```python
from build123d import *

# Parameters (mm, degrees)
BOSS_EXTRUDE1_DEPTH             = 12.7
F_43_0_089_DIAMETER_HOLE1_D     = 2.2606
F_43_0_089_DIAMETER_HOLE1_DEPTH = 25.4
F_43_0_089_DIAMETER_HOLE1_TIP   = 0.679152758
F_43_0_089_DIAMETER_HOLE2_D     = 2.2606
F_43_0_089_DIAMETER_HOLE2_DEPTH = 25.4
F_43_0_089_DIAMETER_HOLE2_TIP   = 0.679152758


with BuildPart() as part:
    # Sketch1 → Boss-Extrude1 (new body)
    with BuildSketch(Plane(origin=(0, 0, 0), x_dir=(0, 0, -1), z_dir=(1, 0, 0))):
        Polygon((0, 0), (0, 12.7), (3.175, 12.7), (3.175, 3.175), (12.7, 3.175), (12.7, 0), align=None)
    extrude(amount=BOSS_EXTRUDE1_DEPTH)

    # #43 (0.089) Diameter Hole1
    with Locations(Plane(origin=(0, 0, -3.175), x_dir=(-1, 0, 0), z_dir=(0, 0, -1))):
        with Locations((-6.35, 7.9375)):
            Hole(F_43_0_089_DIAMETER_HOLE1_D / 2, depth=F_43_0_089_DIAMETER_HOLE1_DEPTH)
            with Locations((0, 0, -(F_43_0_089_DIAMETER_HOLE1_DEPTH + F_43_0_089_DIAMETER_HOLE1_TIP / 2))):  # 118° drill point
                Cone(0, F_43_0_089_DIAMETER_HOLE1_D / 2, F_43_0_089_DIAMETER_HOLE1_TIP, mode=Mode.SUBTRACT)

    # #43 (0.089) Diameter Hole2
    with Locations(Plane(origin=(0, 3.175, 0), x_dir=(1, 0, 0), z_dir=(0, 1, 0))):
        with Locations((6.35, 7.9375)):
            Hole(F_43_0_089_DIAMETER_HOLE2_D / 2, depth=F_43_0_089_DIAMETER_HOLE2_DEPTH)
            with Locations((0, 0, -(F_43_0_089_DIAMETER_HOLE2_DEPTH + F_43_0_089_DIAMETER_HOLE2_TIP / 2))):  # 118° drill point
                Cone(0, F_43_0_089_DIAMETER_HOLE2_D / 2, F_43_0_089_DIAMETER_HOLE2_TIP, mode=Mode.SUBTRACT)


solid = part.part
```
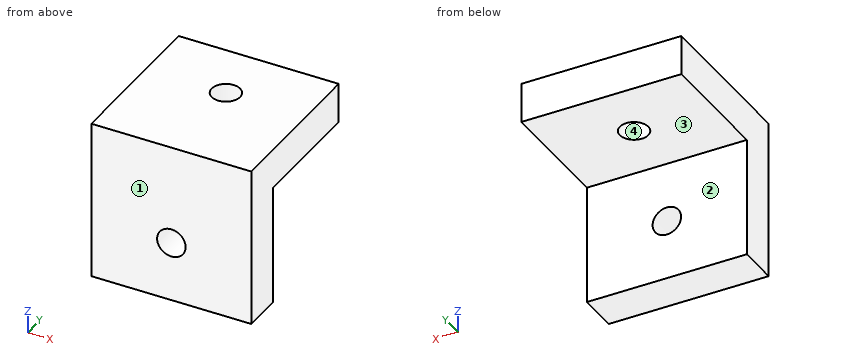
Here's how the part is built. I have some questions about the finished solid (model axes, mm). Face numbers are marked on the shaded views. Round coordinates to 2 decimals unless told otherwise and drop trailing zeros. Write each loop counter-clockwise with the first axis right and the second up, starting at its lowest first coordinate (ties: lowest second). Pieces come first, ordered by that corner, then holes. Notation, with made-up numbers: M -7.75,-7.75 L 27.25,-7.75 A28 ccw 27.25,26.25 Z; hole C 69.25,79 d2. An arc over 180 degrees is marked long. Answer as CSV lines item,"result". Start each with the question number.
1. Suppose I cut it at A-A on x = 6.35. Write out the boundary of the cut face in (y, z) (3 decimals), then the cut area to 3 significant figures.
2. I'm going to push flat-ended pins straight in: pin 1 Ø2 at (x, z) = (3.5, -6) entering from +Y (3 decimals); pin 2 Ø7.5 at (x, y) = (3.5, 9.5) entering from -Z (3 decimals); pin 3 Ø1.4 at (x, z) = (6.35, -7.94) entering from -Y. Where does each tip first touch, or does it pass through?
3. Suppose I cut it at C-C on z = -1.25. Write out the boundary of the cut face in (x, y).
4. Suppose I cut it at D-D on x = 11.5. Write out the boundary of the cut face in (y, z) (3 decimals), then the cut area to 3 significant figures.
5. Thinking about a two-plate mould opening in Y: for the marked faces 1, 2, 3 and 4, which applies, released by +Y, released by -Y, zero draft, split by the parting line, or undercut?
6. Suppose I cut it at B-B on y = 8.25. Write out the boundary of the cut face in (x, z) (3 decimals), then the cut area to 3 significant figures.
7. I need wall thicknesses on probe 1 along Z at (x, y) = (6.35, 1.1); probe 2 along Y at (x, z) = (6.35, -2.5); probe 3 along X at (y, z) = (8, -1.75). Which ranges of each line are inside material? Lowest first, please.
Check result:
1,outline,"M 0,-12.7 L 3.175,-12.7 L 3.175,-9.068 L 0,-9.068 Z; M 0,-6.807 L 3.175,-6.807 L 3.175,-3.175 L 6.807,-3.175 L 6.807,0 L 0,0 Z; M 9.068,-3.175 L 12.7,-3.175 L 12.7,0 L 9.068,0 Z"
1,area,"56.2 mm2"
2,pin 1,"stops at y = 3.175"
2,pin 2,"stops at z = -3.175"
2,pin 3,"passes through"
3,outline,"M 0,0 L 12.7,0 L 12.7,12.7 L 0,12.7 Z; hole C 6.35,7.94 d2.26"
4,outline,"M 0,-12.7 L 3.175,-12.7 L 3.175,-3.175 L 12.7,-3.175 L 12.7,0 L 0,0 Z"
4,area,"70.6 mm2"
5,face 1,"released by -Y"
5,face 2,"released by +Y"
5,face 3,"zero draft"
5,face 4,"undercut"
6,outline,"M 0,-3.175 L 5.264,-3.175 L 5.264,0 L 0,0 Z; M 7.436,-3.175 L 12.7,-3.175 L 12.7,0 L 7.436,0 Z"
6,area,"33.4 mm2"
7,probe 1,"z = -12.7 to -9.07, -6.81 to 0"
7,probe 2,"y = 0 to 6.81, 9.07 to 12.7"
7,probe 3,"x = 0 to 5.22, 7.48 to 12.7"
